Input: part model. Units: mm. Frame: model coordinates. A direction names the side the tool comes from. Coordinates: 2 decimals unless noted, no trailing zeros.
```python
from build123d import *

# Parameters (mm, degrees)
CHANFREIN1_SIZE              = 1
CHANFREIN1_SIZE2             = 5
BOSS_EXTRU_5_DEPTH           = 20
BOSS_EXTRU_5_2_DEPTH         = 20
ENL_V_MAT_EXTRU_2_DEPTH      = 62.559283201
ENL_V_MAT_EXTRU_2_DEPTH_BACK = 62.559283201
BOSS_EXTRU_6_REACH           = 63.559
BOSS_EXTRU_7_REACH           = 63.559
ENL_V_MAT_EXTRU_3_DEPTH      = 45.313661961
ENL_V_MAT_EXTRU_3_DEPTH_BACK = 45.313661961
ENL_V_MAT_EXTRU_4_DEPTH      = 45.313661961
ENL_V_MAT_EXTRU_4_DEPTH_BACK = 4
ESQUISSE16_R                 = 2.35
ENL_V_START                  = -4
ESQUISSE17_R                 = 2.35
ENL_V_MAT_EXTRU_5_DEPTH      = 4


with BuildPart() as part:
    # Esquisse2 → Lissage2 section 0
    with BuildSketch(Plane(origin=(0, 0, 22.8), x_dir=(-1, 0, 0), z_dir=(0, 0, -1))):
        with BuildLine():
            Line((9.60314516, 16.936366798), (5.221189916, 17.907863235))
            Line((5.221189916, 17.907863235), (-5.221189909, 17.907863235))
            Line((-5.221189909, 17.907863235), (-9.535571585, 16.951348119))
            Line((-9.535571585, 16.951348119), (-26.187917597, 3.514391472))
            Line((-26.187917597, 3.514391472), (-26.187917597, -3.605517616))
            Line((-26.187917597, -3.605517616), (-27.687917597, -3.605517616))
            Line((-27.687917597, -3.605517616), (-27.687917597, 4.231455295))
            Line((-27.687917597, 4.231455295), (-10.203724477, 18.339638298))
            Line((-10.203724477, 18.339638298), (-5.385473287, 19.407863235))
            Line((-5.385473287, 19.407863235), (5.385473294, 19.407863235))
            Line((5.385473294, 19.407863235), (10.271298051, 18.324656976))
            Line((10.271298051, 18.324656976), (27.687917597, 4.270999817))
            Line((27.687917597, 4.270999817), (27.687917597, -3.605517616))
            Line((27.687917597, -3.605517616), (26.187917597, -3.605517616))
            Line((26.187917597, -3.605517616), (26.187917597, 3.553935994))
            Line((26.187917597, 3.553935994), (9.60314516, 16.936366798))
        make_face()
    # Esquisse7 → Lissage2 section 1
    with BuildSketch(Plane.XY):
        with BuildLine():
            Line((30.687917597, -5.105517616), (30.687917597, 5.66558294))
            Line((30.687917597, 5.66558294), (11.54003026, 21.116218655))
            Line((11.54003026, 21.116218655), (5.714040045, 22.407863235))
            Line((5.714040045, 22.407863235), (-5.714040052, 22.407863235))
            Line((-5.714040052, 22.407863235), (-11.607603834, 21.101237334))
            Line((-11.607603834, 21.101237334), (-30.687917597, 5.705127462))
            Line((-30.687917597, 5.705127462), (-30.687917597, -5.105517616))
            Line((-30.687917597, -5.105517616), (-29.187917597, -5.105517616))
            Line((-29.187917597, -5.105517616), (-29.187917597, 4.988063639))
            Line((-29.187917597, 4.988063639), (-10.939450943, 19.712947155))
            Line((-10.939450943, 19.712947155), (-5.549756673, 20.907863235))
            Line((-5.549756673, 20.907863235), (5.549756666, 20.907863235))
            Line((5.549756666, 20.907863235), (10.871877368, 19.727928476))
            Line((10.871877368, 19.727928476), (29.187917597, 4.948519118))
            Line((29.187917597, 4.948519118), (29.187917597, -5.105517616))
            Line((29.187917597, -5.105517616), (30.687917597, -5.105517616))
        make_face()
    loft()

    # Chanfrein1
    chanfrein1_edges = [part.edges().sort_by_distance(p)[0] for p in [
        (-27.687917597, 0.3327411, 22.8),
        (-18.979607824, 11.297828397, 22.8),
        (-7.828385673, 18.866260106, 22.8),
        (-4e-09, 19.407863235, 22.8),
        (7.794598882, 18.873750766, 22.8),
        (18.945821037, 11.285546796, 22.8),
        (27.687917597, 0.312968839, 22.8),
    ]]
    chanfrein1_side = [part.faces().sort_by_distance(p)[0] for p in [
        (-7.541966061, 18.007574003, 22.8),
    ]]
    chamfer(chanfrein1_edges, length=CHANFREIN1_SIZE, length2=CHANFREIN1_SIZE2, reference=chanfrein1_side[0])

    # Esquisse12 → Boss.-Extru.6 (add, up to next)
    with BuildSketch(Plane(origin=(21.92, 0, 0), x_dir=(0, 0, -1), z_dir=(1, 0, 0)), mode=Mode.PRIVATE) as boss_extru_6_sk1:
        Polygon((-16.803867762, -4), (-20, -3.789728142), (-20, 4), (0, 4), (0, -4), align=None)
    boss_extru_6_tool1 = extrude(boss_extru_6_sk1.sketch, amount=BOSS_EXTRU_6_REACH, mode=Mode.PRIVATE) - part.part


with BuildPart() as body_2:
    # Esquisse8 → Boss.-Extru.5 (new body)
    with BuildSketch(Plane(origin=(0, 0, 20), x_dir=(-1, 0, 0), z_dir=(0, 0, -1))):
        with BuildLine():
            Line((-21.92, 4), (-21.92, -4))
            ThreePointArc((-21.92, -4), (-17.92, 0), (-21.92, 4))
        make_face()
    extrude(amount=BOSS_EXTRU_5_DEPTH)


with BuildPart() as body_3:
    # Esquisse8 → Boss.-Extru.5 2 (new body)
    with BuildSketch(Plane(origin=(0, 0, 20), x_dir=(-1, 0, 0), z_dir=(0, 0, -1))):
        with BuildLine():
            Line((21.92, 4), (21.92, -4))
            ThreePointArc((21.92, -4), (17.92, 0), (21.92, 4))
        make_face()
    extrude(amount=BOSS_EXTRU_5_2_DEPTH)


with BuildPart() as enl_v_mat_extru_2_tool:
    # Esquisse11 → Enlèv. mat.-Extru.2 (new, two sides: drawn at the far end of the back side and taken through both)
    with BuildSketch(Plane(origin=(21.92, 0, 0), x_dir=(0, 0, -1), z_dir=(1, 0, 0)).offset(-ENL_V_MAT_EXTRU_2_DEPTH_BACK)):
        Polygon((-20, -3.789728142), (-16.803867762, -4), (-20, -4), align=None)
    extrude(amount=ENL_V_MAT_EXTRU_2_DEPTH + ENL_V_MAT_EXTRU_2_DEPTH_BACK)


with BuildPart() as body_2_1:
    add(body_2.part)

    # Enlèv. mat.-Extru.2: cut by enl_v_mat_extru_2_tool
    add(enl_v_mat_extru_2_tool.part, mode=Mode.SUBTRACT)


with BuildPart() as body_3_1:
    add(body_3.part)

    # Enlèv. mat.-Extru.2: cut by enl_v_mat_extru_2_tool
    add(enl_v_mat_extru_2_tool.part, mode=Mode.SUBTRACT)


with BuildPart() as part_1:
    add(part.part)

    add(body_2_1.part)  # Boss.-Extru.6 merges body 2
    add(boss_extru_6_tool1.solids().sort_by_distance((21.92, 0.008271, 9.981196))[0])

    # Esquisse14 → Boss.-Extru.7 (add, up to next)
    with BuildSketch(Plane.ZY.offset(21.92), mode=Mode.PRIVATE) as boss_extru_7_sk1:
        Polygon((0, 4), (20, 4), (20, -3.789728142), (16.803867762, -4), (0, -4), align=None)
    boss_extru_7_tool1 = extrude(boss_extru_7_sk1.sketch, amount=BOSS_EXTRU_7_REACH, mode=Mode.PRIVATE) - part_1.part

    add(body_3_1.part)  # Boss.-Extru.7 merges body 3
    add(boss_extru_7_tool1.solids().sort_by_distance((-21.92, 0.008271, 9.981196))[0])

    # Esquisse15 → Enlèv. mat.-Extru.3 (cut, two sides: drawn at the far end of the back side and taken through both)
    with BuildSketch(Plane(origin=(0, 0, 0), x_dir=(-1, 0, 0), z_dir=(0, 0, -1)).offset(-ENL_V_MAT_EXTRU_3_DEPTH_BACK)):
        with BuildLine():
            ThreePointArc((-18.5, -2.074511991), (-17.92, 0), (-18.5, 2.074511991))
            Line((-18.5, 2.074511991), (-18.5, -2.074511991))
        make_face()
        with BuildLine():
            Line((18.5, -2.074511991), (18.5, 2.074511991))
            ThreePointArc((18.5, 2.074511991), (17.92, 0), (18.5, -2.074511991))
        make_face()
        with BuildLine():
            Line((18.5, 2.074511991), (18.5, 3.295393564))
            ThreePointArc((18.5, 3.295393564), (17.170682287, 0), (18.5, -3.295393564))
            Line((18.5, -3.295393564), (18.5, -2.074511991))
            ThreePointArc((18.5, -2.074511991), (17.92, 0), (18.5, 2.074511991))
        make_face()
    extrude(amount=ENL_V_MAT_EXTRU_3_DEPTH + ENL_V_MAT_EXTRU_3_DEPTH_BACK, mode=Mode.SUBTRACT)

    # Esquisse16 → Enlèv. mat.-Extru.4 (cut, two sides: drawn at the far end of the back side and taken through both)
    with BuildSketch(Plane(origin=(0, 0, 0), x_dir=(-1, 0, 0), z_dir=(0, 0, -1)).offset(-ENL_V_MAT_EXTRU_4_DEPTH_BACK)):
        with Locations(Location((-21.92, 0, 0), (0, 0, 180))):
            Circle(ESQUISSE16_R)
        with Locations(Location((21.92, 0, 0), (0, 0, 180))):
            Circle(ESQUISSE16_R)
    extrude(amount=ENL_V_MAT_EXTRU_4_DEPTH + ENL_V_MAT_EXTRU_4_DEPTH_BACK, mode=Mode.SUBTRACT)

    # Esquisse17 → Enlèv. mat.-Extru.5 (cut)
    with BuildSketch(Plane.XY.offset(20).offset(ENL_V_START)):
        with Locations((-21.92, 0)):
            Circle(ESQUISSE17_R)
        with Locations((21.92, 0)):
            Circle(ESQUISSE17_R)
    extrude(amount=ENL_V_MAT_EXTRU_5_DEPTH, mode=Mode.SUBTRACT)


solid = part_1.part
```
Item 1: Contact query for flat-ended pins moving along their axis: P1, Ø2, axis at x = 26, z = 14.5, coming from the +Y side; P2, Ø4, axis at x = -22, y = 0, coming from the +Z side; P3, Ø2, axis at x = -26, z = 5.5, coming from the +Y side. Output: stop coordinate, or through.
Result:
P1: stops at y = 7.82
P2: stops at z = 16
P3: stops at y = 9.38
Item 2: Reachability of faces 1 (the face through (-19.98, -3.5, 10.14)), 2 (the face through (19.93, 3.47, 10.14)), 3 (the face through (-24.268, -0.103, 2.028)), 4 (the face through (-24.268, 0.103, 17.972)) from +Z, -Z, +X, -X, +Y, -Y: full face, straight path, thin tool, end or side. Return the list, or none.
Result:
face 1: +Z, -Z, -Y
face 2: +Z, -Z
face 3: -Z
face 4: +Z
Item 3: Mould query, pull axis Y, two halves, no side actions, for faces 5 (the face through (23.764, -3.896, 18.38)), 6 (the face through (25, 4, 10)), 7 (the face through (1.3, 18.2, 22.8)). Classes: +Y half, -Y half, draft (parallel to the pull), parting line (faces both ways), or undercut.
Result:
face 5: -Y half
face 6: undercut
face 7: draft
Item 4: Line query: L1, parallel to Y at x = 21.92, z = 18.4 (3 decimals); L2, parallel to Y at x = 21.92, z = 17.3; L3, parallel to Y at x = 19, z = 7.75. Output: solid intervals per line, ascending.
Result:
L1: y = -3.895 to -2.35, 2.35 to 4, 7.702 to 9.485
L2: y = -3.97 to -2.35, 2.35 to 4, 7.89 to 9.82
L3: y = -2.73 to 2.73, 11.86 to 13.79
Item 5: Section query A-A (z = 3). Count the separate pieces of the cut face and the enclosed holes in it, then the cut area to 3 significant figures.
Result:
separate pieces: 1
enclosed holes: 2
area: 257 mm2
